Input: part model. Units: mm. Frame: model coordinates. A direction names the side the tool comes from. Coordinates: 2 decimals unless noted, no trailing zeros. Write each loop counter-clockwise with the first axis right and the second up, starting at its lowest first coordinate (ties: lowest second). Pieces come first, ordered by that corner, then holes.
1) Draft query along Y for faces 1 (the flat face through (-130, 112.702, 464)), 2 (the flat face through (88, -21, 0)), 3 (the flat face through (84, 106.702, 1347)), 4 (the flat face through (-130, -159.298, 1137)). Return one class per face: pulls with the +Y half, pulls with the -Y half, needs draft (parallel to the pull), parting line crosses it, or undercut.
2) Section query A-A (z = 1647). Output: boundary loops of the cut face in (x, y), then the cut area to 3 significant figures.
3) Line query: L1, parallel to Z at x = -168, y = 120; L2, parallel to Z at x = -142.5, y = 74; L3, parallel to Z at x = 183, y = 47. Output: solid intervals per line, ascending.
4) Pin query (flat end, axial travel): pin 1 Ø10 at (x, z) = (42.5, 1761.5) entering from +Y; pin 2 Ø4 at (x, y) = (-118, -79.5) entering from +Z; pin 3 Ø10 at (y, z) = (-163, 1492.5) entering from +X. Return the tip coordinate at first contact, or that it passes through.
5) Set-up query: faces 5 (the flat face through (-269.638, 114, 881)), 6 (the flat face through (-252.638, -24, 464)), 7 (the flat face through (-130, -156.298, 1137)), 8 (the flat face through (-55, -156, 1770)), 9 (the flat face through (-255.638, -24, 1137)). Return all of +Z, -Z, +X, -X, +Y, -Y with unobstructed straight access to the full face (end or side cutting, diameter ignored); none if empty.
6) Section query B-B (y = 38). State how many separate pieces and enclosed holes the cut face has, then the cut area to 3 significant figures.
from build123d import *

# Parameters (mm, degrees)
F0_W      = 500
F0_H      = 300
F0_W_2    = 460
F0_H_2    = 260
F1_DEPTH  = 20
F2_W      = 80
F2_H      = 3
F3_DEPTH  = 260
F4_W      = 80
F4_H      = 3
F5_DEPTH  = 460
F6_W      = 20
F6_H      = 20
F7_DEPTH  = 1340
F8_W      = 20
F8_H      = 20
F9_DEPTH  = 460
F10_W     = 20
F10_H     = 20
F11_DEPTH = 260
F12_W     = 20
F12_H     = 20
F13_DEPTH = 460
F14_W     = 3
F14_H     = 80
F15_DEPTH = 900
F16_W     = 80
F16_H     = 3
F17_DEPTH = 900
F18_W     = 80
F18_H     = 3
F19_DEPTH = 900
F20_W     = 20
F20_H     = 20
F21_DEPTH = 460
F22_W     = 20
F22_H     = 20
F23_DEPTH = 260
F24_W     = 20
F24_H     = 20
F25_DEPTH = 460
F26_W     = 80
F26_H     = 3
F27_DEPTH = 460
F28_W     = 3
F28_H     = 80
F29_DEPTH = 400
F30_W     = 80
F30_H     = 3
F31_DEPTH = 400
F32_W     = 80
F32_H     = 3
F33_DEPTH = 400
F34_W     = 20
F34_H     = 20
F35_DEPTH = 60
F36_W     = 20
F36_H     = 20
F37_DEPTH = 460
F38_W     = 20
F38_H     = 20
F39_DEPTH = 410
F40_W     = 20
F40_H     = 20
F41_DEPTH = 260
F42_W     = 20
F42_H     = 20
F42_W_2   = 19.9999999999
F43_DEPTH = 425
F44_W     = 20
F44_H     = 20
F45_DEPTH = 260
F46_W     = 20
F46_H     = 20
F47_DEPTH = 460


with BuildPart() as f1:
    # F0 (on Top) → F1 (new body)
    with BuildSketch(Plane.XY):
        with Locations((-19.6381509304, -23.2981824888)):
            Rectangle(F0_W, F0_H)
        with Locations((-19.6381509304, -23.2981824888)):
            Rectangle(F0_W_2, F0_H_2, mode=Mode.SUBTRACT)
    extrude(amount=F1_DEPTH)

    # F2 (on face) → F3 (join, through all)
    with BuildSketch(Plane.XZ.offset(-106.7018175112)):
        with Locations((-129.6381509304, 1.5)):
            Rectangle(F2_W, F2_H)
        with Locations((90.3618490696, 1.5)):
            Rectangle(F2_W, F2_H)
    extrude(amount=F3_DEPTH)

    # F4 (on face) → F5 (join, through all)
    with BuildSketch(Plane(origin=(210.3618490696, 0, 0), x_dir=(0, -1, 0), z_dir=(-1, 0, 0))):
        with Locations((-36.7018175112, 18.5)):
            Rectangle(F4_W, F4_H)
        with Locations((83.2981824888, 18.5)):
            Rectangle(F4_W, F4_H)
    extrude(amount=F5_DEPTH)

    # F6 (on face) → F7 (join)
    with BuildSketch(Plane.XY.offset(20)):
        with Locations((-259.6381509304, 116.7018175112)):
            Rectangle(F6_W, F6_H)
        with Locations((-259.6381509304, -163.2981824888)):
            Rectangle(F6_W, F6_H)
        with Locations((220.3618490696, -163.2981824888)):
            Rectangle(F6_W, F6_H)
        with Locations((220.3618490696, 116.7018175112)):
            Rectangle(F6_W, F6_H)
    extrude(amount=F7_DEPTH)

    # F8 (on face) → F9 (join, through all)
    with BuildSketch(Plane(origin=(210.3618490696, 0, 0), x_dir=(0, -1, 0), z_dir=(-1, 0, 0))):
        with Locations((163.2981824888, 930)):
            Rectangle(F8_W, F8_H)
    extrude(amount=F9_DEPTH)

    # F10 (on face) → F11 (join, through all)
    with BuildSketch(Plane(origin=(0, -153.2981824888, 0), x_dir=(-1, 0, 0), z_dir=(0, 1, 0))):
        with Locations((259.6381509304, 930)):
            Rectangle(F10_W, F10_H)
        with Locations((-220.3618490696, 930)):
            Rectangle(F10_W, F10_H)
    extrude(amount=F11_DEPTH)

    # F12 (on face) → F13 (join, through all)
    with BuildSketch(Plane.YZ.offset(-249.6381509304)):
        with Locations((116.7018175112, 930)):
            Rectangle(F12_W, F12_H)
    extrude(amount=F13_DEPTH)

    # F14 (on face) → F15 (join, through all)
    with BuildSketch(Plane.XY.offset(20)):
        with Locations((-254.1381509304, -23.2981824888)):
            Rectangle(F14_W, F14_H)
    extrude(amount=F15_DEPTH)

    # F16 (on face) → F17 (join, through all)
    with BuildSketch(Plane.XY.offset(20)):
        with Locations((90.3618490696, 111.2018175112)):
            Rectangle(F16_W, F16_H)
        with Locations((-129.6381509304, 111.2018175112)):
            Rectangle(F16_W, F16_H)
    extrude(amount=F17_DEPTH)

    # F18 (on face) → F19 (join, through all)
    with BuildSketch(Plane.XY.offset(20)):
        with Locations((-129.6381509304, -157.7981824888)):
            Rectangle(F18_W, F18_H)
        with Locations((90.3618490696, -157.7981824888)):
            Rectangle(F18_W, F18_H)
    extrude(amount=F19_DEPTH)

    # F20 (on face) → F21 (join, through all)
    with BuildSketch(Plane(origin=(210.3618490696, 0, 0), x_dir=(0, -1, 0), z_dir=(-1, 0, 0))):
        with Locations((163.2981824888, 1350)):
            Rectangle(F20_W, F20_H)
    extrude(amount=F21_DEPTH)

    # F22 (on face) → F23 (join, through all)
    with BuildSketch(Plane(origin=(0, -153.2981824888, 0), x_dir=(-1, 0, 0), z_dir=(0, 1, 0))):
        with Locations((-220.3618490696, 1350)):
            Rectangle(F22_W, F22_H)
        with Locations((259.6381509304, 1350)):
            Rectangle(F22_W, F22_H)
    extrude(amount=F23_DEPTH)

    # F24 (on face) → F25 (join, through all)
    with BuildSketch(Plane(origin=(210.3618490696, 0, 0), x_dir=(0, -1, 0), z_dir=(-1, 0, 0))):
        with Locations((-116.7018175112, 1350)):
            Rectangle(F24_W, F24_H)
    extrude(amount=F25_DEPTH)

    # F26 (on face) → F27 (join, through all)
    with BuildSketch(Plane.YZ.offset(-249.6381509304)):
        with Locations((-83.2981824888, 938.5)):
            Rectangle(F26_W, F26_H)
        with Locations((36.7018175112, 938.5)):
            Rectangle(F26_W, F26_H)
    extrude(amount=F27_DEPTH)

    # F28 (on face) → F29 (join, through all)
    with BuildSketch(Plane.XY.offset(940)):
        with Locations((-254.1381509304, -23.2981824888)):
            Rectangle(F28_W, F28_H)
    extrude(amount=F29_DEPTH)

    # F30 (on face) → F31 (join, through all)
    with BuildSketch(Plane.XY.offset(940)):
        with Locations((90.3618490696, -157.7981824888)):
            Rectangle(F30_W, F30_H)
        with Locations((-129.6381509304, -157.7981824888)):
            Rectangle(F30_W, F30_H)
    extrude(amount=F31_DEPTH)

    # F32 (on face) → F33 (join, through all)
    with BuildSketch(Plane.XY.offset(940)):
        with Locations((90.3618490696, 111.2018175112)):
            Rectangle(F32_W, F32_H)
        with Locations((-129.6381509304, 111.2018175112)):
            Rectangle(F32_W, F32_H)
    extrude(amount=F33_DEPTH)

    # F34 (on face) → F35 (join)
    with BuildSketch(Plane(origin=(0, 126.7018175112, 0), x_dir=(-1, 0, 0), z_dir=(0, 1, 0))):
        with Locations((-220.3618490696, 1350)):
            Rectangle(F34_W, F34_H)
        with Locations((259.6381509304, 1350)):
            Rectangle(F34_W, F34_H)
        with Locations((-220.3618490696, 1300)):
            Rectangle(F34_W, F34_H)
        with Locations((259.6381509304, 1300)):
            Rectangle(F34_W, F34_H)
    extrude(amount=F35_DEPTH)

    # F36 (on face) → F37 (join, through all)
    with BuildSketch(Plane(origin=(210.3618490696, 0, 0), x_dir=(0, -1, 0), z_dir=(-1, 0, 0))):
        with Locations((-176.7018175112, 1350)):
            Rectangle(F36_W, F36_H)
    extrude(amount=F37_DEPTH)

    # F38 (on face) → F39 (join)
    with BuildSketch(Plane.XY.offset(1360)):
        with Locations((-259.6381509304, -163.2981824888)):
            Rectangle(F38_W, F38_H)
        with Locations((-259.6381509304, 116.7018175112)):
            Rectangle(F38_W, F38_H)
        with Locations((185.3618490696, 116.7018175112)):
            Rectangle(F38_W, F38_H)
        with Locations((185.3618490696, -163.2981824888)):
            Rectangle(F38_W, F38_H)
    extrude(amount=F39_DEPTH)

    # F40 (on face) → F41 (join, through all)
    with BuildSketch(Plane.XZ.offset(-106.7018175112)):
        with Locations((185.3618490696, 1760)):
            Rectangle(F40_W, F40_H)
    extrude(amount=F41_DEPTH)

    # F42 (on face) → F43 (join, through all)
    with BuildSketch(Plane(origin=(175.3618490696, 0, 0), x_dir=(0, -1, 0), z_dir=(-1, 0, 0))):
        with Locations((-116.7018175112, 1760)):
            Rectangle(F42_W, F42_H)
        with Locations((163.2981824889, 1760)):
            Rectangle(F42_W_2, F42_H)
    extrude(amount=F43_DEPTH)

    # F44 (on face) → F45 (join, through all)
    with BuildSketch(Plane.XZ.offset(-106.7018175112)):
        with Locations((-259.6381509304, 1760)):
            Rectangle(F44_W, F44_H)
    extrude(amount=F45_DEPTH)

    # F46 (on face) → F47 (join, through all)
    with BuildSketch(Plane(origin=(210.3618490696, 0, 0), x_dir=(0, -1, 0), z_dir=(-1, 0, 0))):
        with Locations((-176.7018175112, 1300)):
            Rectangle(F46_W, F46_H)
    extrude(amount=F47_DEPTH)


solid = f1.part
Answer:
1. face 1: pulls with the +Y half
1. face 2: needs draft
1. face 3: undercut
1. face 4: pulls with the -Y half
2. outline: (-269.64, -173.3) - (-249.64, -173.3) - (-249.64, -153.3) - (-269.64, -153.3) - close; (-269.64, 106.7) - (-249.64, 106.7) - (-249.64, 126.7) - (-269.64, 126.7) - close; (175.36, -173.3) - (195.36, -173.3) - (195.36, -153.3) - (175.36, -153.3) - close; (175.36, 106.7) - (195.36, 106.7) - (195.36, 126.7) - (175.36, 126.7) - close
2. area: 1,600 mm2
3. L1: z = 0 to 20, 920 to 940, 1340 to 1360, 1750 to 1770
3. L2: z = 0 to 3, 17 to 20, 937 to 940
3. L3: z = 17 to 20, 937 to 940, 1750 to 1770
4. pin 1: stops at y = 126.7
4. pin 2: stops at z = 940
4. pin 3: stops at x = 195.36
5. face 5: +Z, -Z, -X, +Y, -Y
5. face 6: +X
5. face 7: none
5. face 8: +Z, +X, -X, +Y, -Y
5. face 9: -X
6. separate pieces: 8
6. enclosed holes: 0
6. area: 6,440 mm2
